Here's how the part is built. I have some questions about the finished solid (model axes, mm). A direction names the side the tool comes from. Round coordinates to 2 decimals unless told otherwise and drop trailing zeros. Order: outer loops, then holes, each group sorted by start corner. A loop starts at its lowest first (then second) coordinate and runs counter-clockwise, first axis right, second up.
```python
from build123d import *

# Parameters (mm, degrees)
SKETCH1_W                          = 54
SKETCH1_H                          = 34
BOSS_EXTRUDE1_DEPTH                = 2
SKETCH4_R                          = 1.5
BOSS_EXTRUDE2_DEPTH                = 5
M1_2X0_25_TAPPED_HOLE1_D           = 0.95
M1_2X0_25_TAPPED_HOLE1_DEPTH       = 5
M1_2X0_25_TAPPED_HOLE1_CSINK_D     = 1.25
M1_2X0_25_TAPPED_HOLE1_CSINK_ANGLE = 90
M1_2X0_25_TAPPED_HOLE1_TIP         = 0.285408794


with BuildPart() as part:
    # Sketch1 → Boss-Extrude1 (new body)
    with BuildSketch(Plane(origin=(0, 0, 0), x_dir=(1, 0, 0), z_dir=(0, 1, 0))):
        with Locations((-15.073860766, 22.005565176)):
            Rectangle(SKETCH1_W, SKETCH1_H)
    extrude(amount=BOSS_EXTRUDE1_DEPTH)

    # Sketch4 → Boss-Extrude2 (add)
    with BuildSketch(Plane.XZ):
        with Locations(Location((-40.073860766, -7.005565176, 0), (0, 0, 90))):
            Circle(SKETCH4_R)
        with Locations(Location((9.897863343, -7.006700775, 0), (0, 0, 90))):
            Circle(SKETCH4_R)
        with Locations(Location((9.897863343, -37.006700775, 0), (0, 0, 90))):
            Circle(SKETCH4_R)
        with Locations(Location((-40.073860766, -37.005565176, 0), (0, 0, 90))):
            Circle(SKETCH4_R)
    extrude(amount=BOSS_EXTRUDE2_DEPTH)

    # M1.2x0.25 Tapped Hole1
    with Locations(Plane(origin=(-40.073860766, -5, -7.005565176), x_dir=(0, 0, -1), z_dir=(0, -1, 0))):
        with Locations((0, 0), (30, 0), (0.001135599, 49.971724109), (30.001135599, 49.971724109)):
            CounterSinkHole(M1_2X0_25_TAPPED_HOLE1_D / 2, M1_2X0_25_TAPPED_HOLE1_CSINK_D / 2, depth=M1_2X0_25_TAPPED_HOLE1_DEPTH, counter_sink_angle=M1_2X0_25_TAPPED_HOLE1_CSINK_ANGLE)
            with Locations((0, 0, -(M1_2X0_25_TAPPED_HOLE1_DEPTH + M1_2X0_25_TAPPED_HOLE1_TIP / 2))):  # 118° drill point
                Cone(0, M1_2X0_25_TAPPED_HOLE1_D / 2, M1_2X0_25_TAPPED_HOLE1_TIP, mode=Mode.SUBTRACT)


solid = part.part
```
1. If we section it at B-B, the plane x = -17.5: Write out the boundary of the cut face in (y, z), and give its area (3 significant figures).
Evaluation:
outline: (0, -39.01) - (2, -39.01) - (2, -5.01) - (0, -5.01) - close
area: 68.0 mm2
2. If we section it at A-A, the plane y = -0.75: Write out the boundary of the cut face in (x, z) (3 decimals).
Evaluation:
outline: circle Ø3 at (-40.074, -37.006); circle Ø3 at (-40.074, -7.006); circle Ø3 at (9.898, -37.007); circle Ø3 at (9.898, -7.007); hole circle Ø0.95 at (-40.074, -37.006); hole circle Ø0.95 at (-40.074, -7.006); hole circle Ø0.95 at (9.898, -37.007); hole circle Ø0.95 at (9.898, -7.007)
3. If we mould it in two halves opening along Z, with no side actions, what happens to faces 3 (the flat face through (-40, -5, -6)), 4 (the flat face through (-15, 1, -5.006)), 5 (the cylindrical face through (10.47, -2.46, -5.62))? For each: released by +Z, released by -Z, zero draft, split by the parting line, or undercut.
Evaluation:
face 3: zero draft
face 4: released by +Z
face 5: undercut
4. On a 3-axis mill with a long thin cutter (end or side, diameter ignored), from which of +Z, -Z, +X, -X, +Y, -Y can I reach the whole of each face in a straight line? I mean faces 1 (the flat face through (-42.074, 1, -22)), 2 (the cylindrical face through (10.47, -2.46, -35.62)). Say none if no direction works.
Evaluation:
face 1: +Z, -Z, -X, +Y, -Y
face 2: -Y
5. I need wall thicknesses on probe 1 along Y at (x, z) = (8.5, -10.5); probe 2 along X at (y, z) = (-2.75, -8). Which ranges of each line are inside material? Lowest first, please.
Evaluation:
probe 1: y = 0 to 2
probe 2: x = -41.2 to -38.95, 8.77 to 11.02
6. I'm going to push a flat-ended pin straight in: P1, Ø4, axis at x = -34.5, z = -28, coming from the -Y side. Where does the tip first touch, or does it pass through?
Evaluation:
P1: stops at y = 0
7. If we section it at C-C, the plane z = -22: Write out the boundary of the cut face in (x, y), and give its area (3 significant figures).
Evaluation:
outline: (-42.07, 0) - (11.93, 0) - (11.93, 2) - (-42.07, 2) - close
area: 108 mm2
